Geometry check sheet. Reference: the model listing, model coordinates, mm. A direction names the side the tool comes from. Round coordinates to 2 decimals unless told otherwise and drop trailing zeros. Order: outer loops, then holes, each group sorted by start corner. A loop starts at its lowest first (then second) coordinate and runs counter-clockwise, first axis right, second up. Notation, with made-up numbers: (0.5, 1.5) - (24.5, 1.5) arc R16 cw to (24.5, 32.5) - close; hole circle Ø5 at (2.25, 4.25). An arc over 180 degrees is marked (long way). Use a Markdown table: item, result. Add a question column.
(1) Gauge pin test, flat ends, axial feed: P1, Ø3, axis at y = 9, z = 2.5, coming from the +X side; P2, Ø3, axis at y = -1.5, z = 2, coming from the -X side. Record the tip position at first contact, or that the pin passes through.
(2) Mould release check, pull along Y, two halves, no side actions. Record for faces 1 (the face through (10, 9, 3)), 2 (the face through (-2, 1, 0)), 3 (the face through (2, 37.5, 3)), 4 (the face through (-2, -37.5, 3)): released by +Y, released by -Y, zero draft, split by the parting line, or undercut.
(3) Section check A-A on z = 1.35. Record the boundary of the cut face in (x, y).
(4) Access from +Z, -Z, +X, -X, +Y, -Y to the whole of each face (thin tool, end or side, straight path). Record for faces 5 (the face through (147, 12.5, 3)), 6 (the face through (-150, -25, 3)), 7 (the face through (-147, 12.5, 3)), 8 (the face through (0, 6.5, 3)).
(5) Thickness scan on line 1 along Y through (x, z) = (-86.5, 1.25); line 2 along X through (y, z) = (2, 2.15). Record the ranges inside material, lowest first. Write a range as [from, to].
Solid Edge part; units mm, degrees
sketch "Sketch1" plane through (0, 0, 0) normal (0, 0, 1) x (1, 0, 0)
  line L0 (-150, -37.5) -> (150, -37.5)
  line L1 (150, -37.5) -> (150, -12.5)
  line L2 (144, -12.5) -> (150, -12.5)
  line L3 (144, 12.5) -> (144, -12.5)
  line L4 (150, 12.5) -> (144, 12.5)
  line L5 (150, 12.5) -> (150, 37.5)
  line L6 (150, 37.5) -> (-150, 37.5)
  line L7 (-150, 37.5) -> (-150, 12.5)
  line L8 (-144, 12.5) -> (-150, 12.5)
  line L9 (-144, -12.5) -> (-144, 12.5)
  line L10 (-150, -12.5) -> (-144, -12.5)
  line L11 (-150, -12.5) -> (-150, -37.5)
  dimension "D1" = 144
extrude "Protrusion1" add sketch "Sketch1" along normal blind 6
sketch "Sketch2" plane through (0, 0, 6) normal (0, 0, 1) x (1, 0, 0)
  line L0 (-90, 6.5) -> (-70, 6.5)
  line L1 (-70, 6.5) -> (-70, 12.5)
  line L2 (-70, 12.5) -> (-90, 12.5)
  line L3 (-90, 12.5) -> (-90, 6.5)
  line L4 (-10, 6.5) -> (10, 6.5)
  line L5 (10, 6.5) -> (10, 12.5)
  line L6 (10, 12.5) -> (-10, 12.5)
  line L7 (-10, 12.5) -> (-10, 6.5)
  line L8 (70, 6.5) -> (90, 6.5)
  line L9 (90, 6.5) -> (90, 12.5)
  line L10 (90, 12.5) -> (70, 12.5)
  line L11 (70, 12.5) -> (70, 6.5)
  dimension "D1" = 70
  dimension "D2" = 90
  dimension "D3" = 70
  dimension "D4" = 70
  dimension "D5" = 90
extrude "Cutout1" cut sketch "Sketch2" against normal through all
Check sheet entries:
| question | item | result |
|---|---|---|
| 1 | P1 | stops at x = 144 |
| 1 | P2 | stops at x = -144 |
| 2 | face 1 | undercut |
| 2 | face 2 | zero draft |
| 2 | face 3 | released by +Y |
| 2 | face 4 | released by -Y |
| 3 | outline | (-150, -37.5) - (150, -37.5) - (150, -12.5) - (144, -12.5) - (144, 12.5) - (150, 12.5) - (150, 37.5) - (-150, 37.5) - (-150, 12.5) - (-144, 12.5) - (-144, -12.5) - (-150, -12.5) - close; hole (-90, 6.5) - (-70, 6.5) - (-70, 12.5) - (-90, 12.5) - close; hole (-10, 6.5) - (10, 6.5) - (10, 12.5) - (-10, 12.5) - close; hole (70, 6.5) - (90, 6.5) - (90, 12.5) - (70, 12.5) - close |
| 4 | face 5 | +Z, -Z, +X |
| 4 | face 6 | +Z, -Z, -X, +Y, -Y |
| 4 | face 7 | +Z, -Z, -X |
| 4 | face 8 | +Z, -Z |
| 5 | line 1 | y = [-37.5, 6.5], [12.5, 37.5] |
| 5 | line 2 | x = [-144, 144] |
